Input: part model. Units: mm. Frame: model coordinates. Face numbers are marked on the shaded views. A direction names the side the tool comes from. Round coordinates to 2 decimals unless told otherwise and drop trailing zeros. Write each loop counter-clockwise with the first axis right and the second up, starting at its lowest first coordinate (ties: lowest second). Pieces come first, ordered by that corner, then holes. Notation, with made-up numbers: (14.5, 17) -> (41.5, 17) arc R18 ccw to (41.5, 27) -> close; hole circle Ø2 at (-29.75, 47.25). An arc over 180 degrees is marked (long way). Write item = value, one per line.
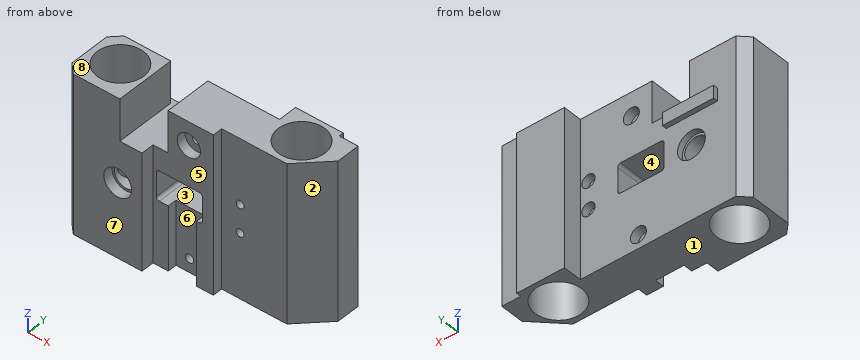
```python
from build123d import *

# Parameters (mm, degrees)
SKETCH1_W           = 158.11
SKETCH1_H           = 108
BOSS_EXTRUDE1_DEPTH = 53.94
SKETCH2_W           = 12.86
SKETCH2_H           = 108
CUT_EXTRUDE1_DEPTH  = 3.2
SKETCH3_W           = 112.68
SKETCH3_H           = 108
CUT_EXTRUDE2_DEPTH  = 12.91
SKETCH4_W           = 104.72
SKETCH4_H           = 108
CUT_EXTRUDE3_DEPTH  = 8.92
SKETCH5_W           = 63.51
SKETCH5_H           = 189.255900931
CUT_EXTRUDE4_DEPTH  = 15.62
SKETCH6_W           = 25.37
SKETCH6_H           = 28.45
CUT_EXTRUDE5_DEPTH  = 199.927865569
SKETCH7_W           = 31.55
SKETCH7_H           = 20.36
CUT_EXTRUDE6_DEPTH  = 196.82194208
FILLET1_R           = 2
CHAMFER1_SIZE       = 6.48
CHAMFER2_SIZE       = 18.99
HOLE1_D             = 31.75
SKETCH10_W          = 19.431
SKETCH10_H          = 43.86
CUT_EXTRUDE7_DEPTH  = 6.223
SKETCH11_R          = 9.525
CUT_EXTRUDE10_DEPTH = 6.6802
SKETCH12_R          = 7.9375
CUT_EXTRUDE11_DEPTH = 198.221349747
CUT_EXTRUDE12_START = -3.9624
SKETCH13_R          = 9.525
CUT_EXTRUDE12_DEPTH = 3.9624
SKETCH14_W          = 34.9758
SKETCH14_H          = 8.763
BOSS_EXTRUDE2_DEPTH = 3.175
HOLE2_D             = 5.7785
HOLE2_CBORE_D       = 10.922
HOLE2_CBORE_DEPTH   = 6.2738
SKETCH18_R          = 7.9375
CUT_EXTRUDE13_DEPTH = 6.35
HOLE3_D             = 5.334
HOLE3_CBORE_D       = 9.0424
HOLE3_CBORE_DEPTH   = 5.334


with BuildPart() as part:
    # Sketch1 → Boss-Extrude1 (new body)
    with BuildSketch(Plane(origin=(0, 0, 0), x_dir=(1, 0, 0), z_dir=(0, 1, 0))):
        with Locations((79.055, -54)):
            Rectangle(SKETCH1_W, SKETCH1_H)
    extrude(amount=BOSS_EXTRUDE1_DEPTH)

    # Sketch2 → Cut-Extrude1 (cut)
    with BuildSketch(Plane(origin=(0, 53.94, 0), x_dir=(-1, 0, 0), z_dir=(0, 1, 0))):
        with Locations((-151.68, 54)):
            Rectangle(SKETCH2_W, SKETCH2_H)
    extrude(amount=-CUT_EXTRUDE1_DEPTH, mode=Mode.SUBTRACT)

    # Sketch3 → Cut-Extrude2 (cut)
    with BuildSketch(Plane(origin=(0, 53.94, 0), x_dir=(-1, 0, 0), z_dir=(0, 1, 0))):
        with Locations((-56.34, 54)):
            Rectangle(SKETCH3_W, SKETCH3_H)
    extrude(amount=-CUT_EXTRUDE2_DEPTH, mode=Mode.SUBTRACT)

    # Sketch4 → Cut-Extrude3 (cut)
    with BuildSketch(Plane.XZ):
        with Locations((105.75, 54)):
            Rectangle(SKETCH4_W, SKETCH4_H)
    extrude(amount=-CUT_EXTRUDE3_DEPTH, mode=Mode.SUBTRACT)

    # Sketch5 → Cut-Extrude4 (cut)
    with BuildSketch(Plane.XZ):
        with Locations((126.355, 87.843662975)):
            Rectangle(SKETCH5_W, SKETCH5_H)
    extrude(amount=-CUT_EXTRUDE4_DEPTH, mode=Mode.SUBTRACT)

    # Sketch6 → Cut-Extrude5 (cut, through all)
    with BuildSketch(Plane(origin=(0, 53.94, 0), x_dir=(-1, 0, 0), z_dir=(0, 1, 0))):
        with Locations((-50.955, 93.775)):
            Rectangle(SKETCH6_W, SKETCH6_H)
    extrude(amount=-CUT_EXTRUDE5_DEPTH, mode=Mode.SUBTRACT)

    # Sketch7 → Cut-Extrude6 (cut, through all)
    with BuildSketch(Plane(origin=(0, 41.03, 0), x_dir=(1, 0, 0), z_dir=(0, 1, 0))):
        with Locations((71.375, -54.04)):
            Rectangle(SKETCH7_W, SKETCH7_H)
    extrude(amount=-CUT_EXTRUDE6_DEPTH, mode=Mode.SUBTRACT)

    # Fillet1
    fillet1_edges = [part.edges().sort_by_distance(p)[0] for p in [
        (55.6, 24.975, 64.22),
        (55.6, 24.975, 43.86),
        (87.15, 24.975, 43.86),
        (87.15, 24.975, 64.22),
    ]]
    fillet(fillet1_edges, radius=FILLET1_R)

    # Chamfer1
    chamfer1_edges = [part.edges().sort_by_distance(p)[0] for p in [
        (0, 41.03, 54),
        (0, 0, 54),
    ]]
    chamfer(chamfer1_edges, length=CHAMFER1_SIZE)

    # Chamfer2
    chamfer2_edges = [part.edges().sort_by_distance(p)[0] for p in [
        (158.11, 15.62, 54),
    ]]
    chamfer(chamfer2_edges, length=CHAMFER2_SIZE)

    # Hole1 (through all)
    with Locations(Plane(origin=(0, 0, 0), x_dir=(-1, 0, 0), z_dir=(0, 0, -1))):
        with Locations((-19.812, 22.225), (-132.7862, 35.017)):
            Hole(HOLE1_D / 2)

    # Sketch10 → Cut-Extrude7 (cut)
    with BuildSketch(Plane.XZ.offset(-8.92)):
        with Locations((73.5195, 21.93)):
            Rectangle(SKETCH10_W, SKETCH10_H)
    extrude(amount=-CUT_EXTRUDE7_DEPTH, mode=Mode.SUBTRACT)

    # Sketch11 → Cut-Extrude10 (cut)
    with BuildSketch(Plane.XZ):
        with Locations(Location((36.83, 50.8, 0), (0, 0, 270))):
            Circle(SKETCH11_R)
    extrude(amount=-CUT_EXTRUDE10_DEPTH, mode=Mode.SUBTRACT)

    # Sketch12 → Cut-Extrude11 (cut, through all)
    with BuildSketch(Plane.XZ.offset(-6.6802)):
        with Locations(Location((36.83, 50.8, 0), (0, 0, 270))):
            Circle(SKETCH12_R)
    extrude(amount=-CUT_EXTRUDE11_DEPTH, mode=Mode.SUBTRACT)

    # Sketch13 → Cut-Extrude12 (cut)
    with BuildSketch(Plane(origin=(0, 41.03, 0), x_dir=(-1, 0, 0), z_dir=(0, 1, 0)).offset(CUT_EXTRUDE12_START)):
        with Locations(Location((-36.83, 50.8, 0), (0, 0, 270))):
            Circle(SKETCH13_R)
    extrude(amount=CUT_EXTRUDE12_DEPTH, mode=Mode.SUBTRACT)

    # Sketch14 → Boss-Extrude2 (add)
    with BuildSketch(Plane(origin=(0, 41.03, 0), x_dir=(1, 0, 0), z_dir=(0, 1, 0))):
        with Locations((36.5379, -75.1685)):
            Rectangle(SKETCH14_W, SKETCH14_H)
    extrude(amount=BOSS_EXTRUDE2_DEPTH)

    # Hole2 (through all)
    with Locations(Plane(origin=(0, 41.03, 0), x_dir=(-1, 0, 0), z_dir=(0, 1, 0))):
        with Locations((-73.025, 9.398), (-77.864, 91.998)):
            CounterBoreHole(HOLE2_D / 2, HOLE2_CBORE_D / 2, HOLE2_CBORE_DEPTH)

    # Sketch18 → Cut-Extrude13 (cut)
    with BuildSketch(Plane.XZ.offset(-8.92)):
        with Locations(Location((77.864, 91.998, 0), (0, 0, 270))):
            Circle(SKETCH18_R)
    extrude(amount=-CUT_EXTRUDE13_DEPTH, mode=Mode.SUBTRACT)

    # Hole3 (through all)
    with Locations(Plane(origin=(0, 41.03, 0), x_dir=(-1, 0, 0), z_dir=(0, 1, 0))):
        with Locations((-107.2084, 44.5262), (-107.2084, 63.5762)):
            CounterBoreHole(HOLE3_D / 2, HOLE3_CBORE_D / 2, HOLE3_CBORE_DEPTH)


solid = part.part
```
1) Cut plane D-D (x = 137). Return the cut outline in (y, z).
Solutions:
outline = (15.62, 0) -> (19.71, 0) -> (19.71, 108) -> (15.62, 108) -> close; (50.32, 0) -> (53.94, 0) -> (53.94, 108) -> (50.32, 108) -> close
2) First-contact query: P1, Ø2.5, axis at x = 36.5, z = 76, coming from the +Y side (3 decimals); P2, Ø12, axis at x = 26.5, y = 31.5, coming from the +Z side; P3, Ø8.5, axis at x = 107.21, z = 44.53, coming from the +Y side; P4, Ø14.5, axis at x = 77.864, z = 91.998, coming from the +Y side. Flat tips, straight axial feed; report the tip coordinate or a pass-through.
Solutions:
P1 = 44.205
P2 = 108
P3 = 35.7
P4 = 41.03
3) Access query for the marked faces 4, 5, 6, 7 and 8. Directions: +Z, -Z, +X, -X, +Y, -Y. A direction counts if a zero-diameter tool reaches every point of the face in a straight line with its end or side. Return the directions, or none.
Solutions:
face_4 = +Y, -Y
face_5 = +Z, -Z, +X, -Y
face_6 = -Z, -Y
face_7 = +Z, -Z, +X, -X, -Y
face_8 = +Z, +X, -X, +Y, -Y
4) Line query: L1, parallel to Z at x = 63, y = 18; L2, parallel to X at y = 36.5, z = 98; L3, parallel to X at y = 36, z = 48. Output: solid intervals per line, ascending. Write a range as from..to.
Solutions:
L1 = 0..43.86, 64.22..79.55
L2 = 1.95..12.87, 26.76..38.27, 63.64..116.98, 148.59..158.11
L3 = 1.45..11.92, 27.7..29.4, 44.26..55.6, 87.15..104.31, 110.1..116.94, 148.63..158.11
5) Draft query along Z for the marked faces 1, 2 and 3. Return one class per face: +Z half, -Z half, draft (parallel to the pull), parting line (faces both ways), or undercut.
Solutions:
face_1 = -Z half
face_2 = draft
face_3 = undercut
6) Cut plane B-B (x = 17). Return the cut outline in (y, z), and give its area (3 significant figures).
Solutions:
outline = (0, 0) -> (6.6, 0) -> (6.6, 108) -> (0, 108) -> close; (37.85, 0) -> (41.03, 0) -> (41.03, 108) -> (37.85, 108) -> close
area = 1,060 mm^2
7) Cut plane A-A (z = 50.8). Count the separate pieces of the cut face and the enclosed holes in it, and give its area (3 significant figures).
Solutions:
separate_pieces = 3
enclosed_holes = 1
area = 2,290 mm^2
